from build123d import *

# Parameters (mm, degrees)
EXTRUDE1_DEPTH = 15


with BuildPart() as part:
    # Sketch1 → Extrude1 (new body)
    with BuildSketch(Plane(origin=(0, 0, 0), x_dir=(1, 0, 0), z_dir=(0, 1, 0))):
        Polygon((69.389262615, -95.450849719), (116.942088429, -80), (116.942088429, -30), (69.389262615, -14.549150281), (40, -55), align=None)
    extrude(amount=EXTRUDE1_DEPTH)

    # Sketch3 → Loft1 section 0
    with BuildSketch(Plane(origin=(0, 15, 0), x_dir=(1, 0, 0), z_dir=(0, 1, 0)), mode=Mode.PRIVATE) as loft1_s0:
        Polygon((69.389262615, -95.450849719), (40, -55), (69.389262615, -14.549150281), (116.942088429, -30), (116.942088429, -80), align=None)
    loft([loft1_s0.sketch, Vertex(82.532540418, 65, 55)])


solid = part.part
The listing builds one solid part. Answer for the finished solid, in the listing's coordinates (mm). Give positions to 0.01 mm unless a question says otherwise; leave off trailing zeros. Order: outer loops, then holes, each group sorted by start corner. A loop starts at its lowest first (then second) coordinate and runs counter-clockwise, first axis right, second up. Notation, with made-up numbers: (80.25, 77.25) - (89.25, 77.25) arc R18 ccw to (89.25, 101.25) - close; hole circle Ø8 at (-19.75, 60). An arc over 180 degrees is marked (long way). Use one line per item in the form item = value.
1) Find section C-C on z = 39.5. Determine the outline of the cut face in (x, y).
Verdict:
outline = (51.26, 0) - (116.94, 0) - (116.94, 15) - (103.87, 34) - (77.5, 45.84) - (51.26, 15) - close
2) Find section A-A on x = 79.5. Determine the outline of the cut face in (y, z).
Verdict:
outline = (0, 17.83) - (15, 17.83) - (53.46, 45.67) - (61.44, 55) - (53.46, 64.33) - (15, 92.17) - (0, 92.17) - close
3) Each of these flat-tipped pins is pushed along its axis until it touches: pin 1 (3 mm diameter, centred on y = 19.5, z = 71.5, fed in from +X); pin 2 (6 mm diameter, centred on y = 27, z = 63.5, fed in from -X); pin 3 (3 mm diameter, centred on x = 81, z = 60, fed in from +Y); pin 4 (1 mm diameter, centred on x = 62, z = 50.5, fed in from -Y). Where does it stop, or does it pass through?
Verdict:
pin_1 = 114.88
pin_2 = 53.03
pin_3 = 60.61
pin_4 = 0
4) Find section B-B on y = 10.5. Determine the outline of the cut face in (x, z).
Verdict:
outline = (40, 55) - (69.39, 14.55) - (116.94, 30) - (116.94, 80) - (69.39, 95.45) - close
5) Consider probe 1 along Z at (x, y) = (92, 35); probe 2 along Y at (x, z) = (107.5, 83); probe 3 along Z at (x, y) = (74, 15). Determine where each line is inside the solid, lowest interval first. Write a range as [from, to].
Verdict:
probe_1 = [36.37, 73.63]
probe_2 = [0, 15.09]
probe_3 = [16.05, 93.95]
6) Find section D-D on x = 105.5. Determine the outline of the cut face in (y, z).
Verdict:
outline = (0, 26.28) - (15, 26.28) - (31.63, 38.31) - (31.63, 71.69) - (15, 83.72) - (0, 83.72) - close
